```python
from build123d import *

# Parameters (mm, degrees)
F0_R     = 1.6
F1_DEPTH = 2.3
F2_R     = 5
F3_DEPTH = 7.7
F5_DEPTH = 26.3
F6_R     = 1
F7_DEPTH = 6
F8_SIZE  = 1


with BuildPart() as f1:
    # F0 (on Top) → F1 (new body)
    with BuildSketch(Plane.XY):
        with BuildLine():
            Line((-3, 5.765), (-10.043565, 3.861473))
            ThreePointArc((-10.043565, 3.861473), (-13, 0), (-10.043565, -3.861473))
            Line((-10.043565, -3.861473), (-3, -5.765))
            Line((-3, -5.765), (0, -5.765))
            Line((0, -5.765), (3, -5.765))
            Line((3, -5.765), (10.043565, -3.861473))
            ThreePointArc((10.043565, -3.861473), (13, 0), (10.043565, 3.861473))
            Line((10.043565, 3.861473), (3, 5.765))
            Line((3, 5.765), (0, 5.765))
            Line((0, 5.765), (-3, 5.765))
        make_face()
        with Locations((-9, 0)):
            Circle(F0_R, mode=Mode.SUBTRACT)
        with Locations((9, 0)):
            Circle(F0_R, mode=Mode.SUBTRACT)
    extrude(amount=-F1_DEPTH)

    # F2 (on face) → F3 (join)
    with BuildSketch(Plane(origin=(0, 0, -2.3), x_dir=(1, 0, 0), z_dir=(0, 0, -1))):
        Circle(F2_R)
    extrude(amount=F3_DEPTH)

    # F4 (on face) → F5 (join)
    with BuildSketch(Plane(origin=(0, 0, -10), x_dir=(1, 0, 0), z_dir=(0, 0, -1))):
        with BuildLine():
            Line((6.5, -5), (6.5, 5))
            Line((6.5, 5), (0, 5))
            ThreePointArc((0, 5), (3.535534, 3.535534), (5, 0))
            ThreePointArc((5, 0), (3.535534, -3.535534), (0, -5))
            Line((0, -5), (6.5, -5))
        make_face()
        with BuildLine():
            ThreePointArc((0, -5), (-5, 0), (0, 5))
            Line((0, 5), (-6.5, 5))
            Line((-6.5, 5), (-6.5, -5))
            Line((-6.5, -5), (0, -5))
        make_face()
        with BuildLine():
            ThreePointArc((5, 0), (3.535534, 3.535534), (0, 5))
            ThreePointArc((0, 5), (-5, 0), (0, -5))
            ThreePointArc((0, -5), (3.535534, -3.535534), (5, 0))
        make_face()
    extrude(amount=F5_DEPTH)

    # F6 (on face) → F7 (join)
    with BuildSketch(Plane(origin=(0, 0, -36.3), x_dir=(1, 0, 0), z_dir=(0, 0, -1))):
        Circle(F6_R)
    extrude(amount=F7_DEPTH)

    # F8
    f8_edges = [f1.edges().sort_by_distance(p)[0] for p in [
        (-1, 0, -42.3),
    ]]
    chamfer(f8_edges, length=F8_SIZE)


solid = f1.part
```
The model under review builds one solid part; all positions refer to its coordinate system, in mm. A direction names the side the tool comes from. Round coordinates to 2 decimals unless told otherwise and drop trailing zeros. Order: outer loops, then holes, each group sorted by start corner. A loop starts at its lowest first (then second) coordinate and runs counter-clockwise, first axis right, second up. Notation, with made-up numbers: M -8.5,-39.5 L 16.5,-39.5 A30 cw 16.5,-4.5 Z; hole C 50.25,21.5 d8. An arc over 180 degrees is marked long. Use a Markdown table: item, result.
1) Insertion check: pin 1 (3 mm diameter, centred on y = 0.5, z = -20, fed in from -X); pin 2 (3.5 mm diameter, centred on x = 9, y = 0, fed in from -Z); pin 3 (6.5 mm diameter, centred on x = 2, z = -17, fed in from +Y). Each pin has a flat end and moves straight along its axis. Give the tip position at first contact, or say it passes through.
Report:
| item | result |
|---|---|
| pin 1 | x = -6.5 |
| pin 2 | z = -2.3 |
| pin 3 | y = 5 |
2) Wall thickness on line 1 along Z through (x, y) = (-3, -4.75); line 2 along Y through (x, z) = (-9, -1.55); line 3 along Z through (x, y) = (-4, -0.25): over which ranges is each line inside the solid? List them lowest first. Write a range as [from, to].
Report:
| item | result |
|---|---|
| line 1 | [-36.3, -10], [-2.3, 0] |
| line 2 | [-4.14, -1.6], [1.6, 4.14] |
| line 3 | [-36.3, 0] |
3) Consider section C-C (y = -3.25). Write out the cut boundary in (x, z), then the cut area to 3 significant figures.
Report:
| item | result |
|---|---|
| outline | M -11.33,-2.3 L -3.8,-2.3 L -3.8,-10 L -6.5,-10 L -6.5,-36.3 L 6.5,-36.3 L 6.5,-10 L 3.8,-10 L 3.8,-2.3 L 11.33,-2.3 L 11.33,0 L -11.33,0 Z |
| area | 453 mm^2 |
4) Consider section D-D (x = 2.5). Write out the cut boundary in (y, z) (3 decimals), then the cut area to 3 significant figures.
Report:
| item | result |
|---|---|
| outline | M -5.765,-2.3 L -4.33,-2.3 L -4.33,-10 L -5,-10 L -5,-36.3 L 5,-36.3 L 5,-10 L 4.33,-10 L 4.33,-2.3 L 5.765,-2.3 L 5.765,0 L -5.765,0 Z |
| area | 356 mm^2 |
5) Consider section A-A (x = 9). Write out the cut boundary in (y, z), then the cut area to 3 significant figures.
Report:
| item | result |
|---|---|
| outline | M -4.14,-2.3 L -1.6,-2.3 L -1.6,0 L -4.14,0 Z; M 1.6,-2.3 L 4.14,-2.3 L 4.14,0 L 1.6,0 Z |
| area | 11.7 mm^2 |
6) Draft analysis for pull direction Y (two halves, no side actions). For faces 1 (the face through (-10.6, 0.07, -1.13)), 2 (the face through (-1.08, 4.88, -6.1)), 3 (the face through (-6.472, 4.827, -1.134)), 4 (the face through (7.4, 0.07, -1.13)), state which applies: released by +Y, released by -Y, zero draft, split by the parting line, or undercut.
Report:
| item | result |
|---|---|
| face 1 | undercut |
| face 2 | split by the parting line |
| face 3 | released by +Y |
| face 4 | undercut |
7) Consider section B-B (z = -29.5). Write out the cut boundary in (x, y).
Report:
| item | result |
|---|---|
| outline | M -6.5,-5 L 6.5,-5 L 6.5,5 L -6.5,5 Z |
8) Tool access review of faces 5 (the face through (0, 1, -39)), 6 (the face through (-5.5, -0.1, -10)), 7 (the face through (-6.5, 0, -23)), 8 (the face through (0, 5, -23)): name each direction out of +Z, -Z, +X, -X, +Y, -Y from which nothing blocks a thin tool from reaching the whole face with its end or side.
Report:
| item | result |
|---|---|
| face 5 | -Z |
| face 6 | -X |
| face 7 | -Z, -X, +Y, -Y |
| face 8 | -Z, +X, -X, +Y |
